Model file for the job. Use its own axes, mm. A direction names the side the tool comes from. Give positions to 0.01 mm unless a question says otherwise; leave off trailing zeros. Loops run counter-clockwise (first coordinate to the right, second up) from the corner with the lowest first, then second, coordinate; pieces in that order, holes last. Notation, with made-up numbers: (73, 6) - (109, 6) arc R21 ccw to (109, 10) - close; hole circle Ø8 at (-35.5, 84). An arc over 180 degrees is marked (long way). Use a Markdown table: item, result.
from build123d import *

# Parameters (mm, degrees)
F1_DEPTH = 22
F2_DEPTH = 10
F3_R     = 9.5
F4_DEPTH = 2.5
F5_R     = 1.35
F5_W     = 18.2
F5_H     = 3
F6_DEPTH = 8


with BuildPart() as f1:
    # F0 (on Top) → F1 (new body)
    with BuildSketch(Plane.XY):
        Polygon((0, 21.5), (0, 0), (7.8253600367, 0), align=None)
    extrude(amount=F1_DEPTH)

    # F2 (add): a face of the model
    f2_faces = [f1.faces().sort_by_distance(p)[0] for p in [
        (3.9126800184, 10.75, 11),
    ]]
    extrude(f2_faces, amount=F2_DEPTH)

    # F3 (on face) → F4 (cut)
    with BuildSketch(Plane(origin=(0, 0, 0), x_dir=(0, -1, 0), z_dir=(-1, 0, 0))):
        with Locations((-10.75, 11)):
            Circle(F3_R)
    extrude(amount=-F4_DEPTH, mode=Mode.SUBTRACT)

    # F5 (on face) → F6 (cut)
    with BuildSketch(Plane(origin=(16.306893012, 5.9352236697, 0), x_dir=(-0.3420201433, 0.9396926208, 0), z_dir=(0.9396926208, 0.3420201433, 0))):
        with Locations((0.6633913469, 17.24)):
            Circle(F5_R)
        with Locations((17.6633913469, 4.64)):
            Circle(F5_R)
        with Locations((11.1033913469, 20.5)):
            Rectangle(F5_W, F5_H)
    extrude(amount=-F6_DEPTH, mode=Mode.SUBTRACT)


solid = f1.part
(1) 3-axis set-ups, long thin cutter, end or side, ignore diameter. For faces 5 (the flat face through (4.633, 23.186, 10.846)), 6 (the flat face through (5.035, 13.513, 20.521)), 7 (the flat face through (2.755, 19.779, 4.659)): which of +Z, -Z, +X, -X, +Y, -Y reach the whole face in a straight line?
Computed:
| item | result |
|---|---|
| face 5 | +Z, -Z, -X, +Y |
| face 6 | +Z, +Y |
| face 7 | none |
(2) Pin check, flat tips, straight feed: P1, Ø2, axis at y = 19, z = 10.5, coming from the +X side; P2, Ø5, axis at y = 13.5, z = 7, coming from the -X side; P3, Ø5, axis at x = 3.5, z = 7, coming from the +Y side. Stop position of each tip, or through.
Computed:
| item | result |
|---|---|
| P1 | x = 11.92 |
| P2 | x = 2.5 |
| P3 | y = 23.68 |
(3) Slice it at B-B, the plane y = 10.75. Write the cut outline in (x, z).
Computed:
| item | result |
|---|---|
| outline | (0, 0) - (14.55, 0) - (14.55, 19) - (6.04, 19) - (6.04, 22) - (0, 22) - (0, 20.5) - (2.5, 20.5) - (2.5, 1.5) - (0, 1.5) - close |
(4) Mould opens along Y. For faces 1 (the cylindrical face through (1.23, 17.75, 17.42)), 2 (the flat face through (2.5, 11, 11)), 3 (the flat face through (6, 9, 22)), 4 (the flat face through (4, 0, 11)) say: pulls with the +Y half, pulls with the -Y half, needs draft (parallel to the pull), parting line crosses it, or undercut.
Computed:
| item | result |
|---|---|
| face 1 | undercut |
| face 2 | undercut |
| face 3 | needs draft |
| face 4 | pulls with the -Y half |
(5) Slice it at D-D, the plane z = 18. Write the cut outline in (x, y).
Computed:
| item | result |
|---|---|
| outline | (0, 0) - (7.83, 0) - (17.22, 3.42) - (16.46, 5.51) - (8.94, 2.77) - (8.18, 4.87) - (15.7, 7.61) - (9.4, 24.92) - (0, 21.5) - (0, 17.17) - (2.5, 17.17) - (2.5, 4.33) - (0, 4.33) - close |
(6) Slice it at C-C, the plane z = 2.5. Write the cut outline in (x, y).
Computed:
| item | result |
|---|---|
| outline | (0, 0) - (7.83, 0) - (17.22, 3.42) - (9.4, 24.92) - (0, 21.5) - (0, 14.99) - (2.5, 14.99) - (2.5, 6.51) - (0, 6.51) - close |
(7) Slice it at A-A, the plane z = 11. Write the cut outline in (x, y).
Computed:
| item | result |
|---|---|
| outline | (0, 0) - (7.83, 0) - (17.22, 3.42) - (9.4, 24.92) - (0, 21.5) - (0, 20.25) - (2.5, 20.25) - (2.5, 1.25) - (0, 1.25) - close |
(8) Drill centre lines: probe 1 along Z at (x, y) = (1.85, 10.75); probe 2 along Z at (x, y) = (3.5, 20.25); probe 3 along Y at (x, z) = (6.25, 4). Where is each one in solid material? Low to high. Write a range as [from, to].
Computed:
| item | result |
|---|---|
| probe 1 | [0, 1.5], [20.5, 22] |
| probe 2 | [0, 3.3], [5.98, 19] |
| probe 3 | [0, 19.81], [22.34, 23.77] |
